Check sheet for the modelled part. Datum: model origin and axes. Units: mm. A direction names the side the tool comes from. Round coordinates to 2 decimals unless told otherwise and drop trailing zeros. Loops run counter-clockwise (first coordinate to the right, second up) from the corner with the lowest first, then second, coordinate; pieces in that order, holes last. Notation, with made-up numbers: M 79,11 L 127,11 A7 ccw 127,23 Z; hole C 81,40.25 d8. An arc over 180 degrees is marked long. Write item = value, one per line. Start each with the question number.
(1) Scan lines: L1, parallel to Y at x = 9, z = 17.5; L2, parallel to Y at x = 6.5, z = 6.5; L3, parallel to Y at x = 0, z = 11. Record each from-to range of solid material in increasing order. Write a range as from..to.
(2) Cross-section at D-D on x = 0. Record the boundary of the cut face in (y, z), plus the area to 3 significant figures.
(3) Cross-section at B-B on y = 15. Record the boundary of the cut face in (x, z), plus the area to 3 significant figures.
(4) Mould release check, pull along X, two halves, no side actions. Record for faces 4 (the face through (26.805, 3.237, 11.586)), 5 (the face through (3.4, 16.4, 11.6)), 6 (the face through (-16.2, 21.6, 11.6)): pulls with the +X half, pulls with the -X half, needs draft (parallel to the pull), parting line crosses it, or undercut.
(5) Set-up check for faces 1 (the face through (-3.399, -16.354, 11.586)), 2 (the face through (12.431, -11.115, 11.586)), 3 (the face through (-16.33, 1.26, 11.59)): record each of +Z, -Z, +X, -X, +Y, -Y from which the full face is reachable in a straight line by a thin tool's end or side.
(6) Go/stop test with flat-tipped pins: P1, Ø2.5, axis at x = 0, y = 0, coming from the +Z side; P2, Ø6, axis at x = -6.5, z = 5, coming from the -Y side; P3, Ø1, axis at x = 16, z = 20, coming from the -Y side; P4, Ø2, axis at x = 12.5, z = 19.5, coming from the +Y side. Record where each tip stops, or that it passes through.
(7) Cross-section at A-A on z = 6.5. Record the boundary of the cut face in (x, y).
(8) Cross-section at C-C on x = 10. Record the boundary of the cut face in (y, z), plus the area to 3 significant figures.
from build123d import *

# Parameters (mm, degrees)
EXTRUDE_1_DEPTH          = 23.5
CUT_EXTRUDE_1_DEPTH      = 45.211198656
CUT_EXTRUDE_1_DEPTH_BACK = 45.211198656
SKETCH_2_R               = 2


with BuildPart() as part:
    # 草图1 → 凸台-拉伸1 (new body)
    with BuildSketch(Plane.XY):
        with BuildLine():
            Line((-18.74404726, 19.433494084), (-5.953134221, 2.483458779))
            Line((-5.953134221, 2.483458779), (-27, 0))
            ThreePointArc((-27, 0), (-26.799738116, -3.282382812), (-26.201923191, -6.516074055))
            Line((-26.201923191, -6.516074055), (-5.228535388, -3.928299208))
            Line((-5.228535388, -3.928299208), (-13.5, -23.382685902))
            ThreePointArc((-13.5, -23.382685902), (-10.557242158, -24.850445429), (-7.457875931, -25.949568139))
            Line((-7.457875931, -25.949568139), (0.77550929, -6.485913341))
            Line((0.77550929, -6.485913341), (13.5, -23.382685902))
            ThreePointArc((13.5, -23.382685902), (16.242495958, -21.568062617), (18.74404726, -19.433494084))
            Line((18.74404726, -19.433494084), (5.938212824, -2.560395934))
            Line((5.938212824, -2.560395934), (27, 0))
            ThreePointArc((27, 0), (26.799738116, 3.282382812), (26.201923191, 6.516074055))
            Line((26.201923191, 6.516074055), (5.200951411, 3.927966656))
            Line((5.200951411, 3.927966656), (13.5, 23.382685902))
            ThreePointArc((13.5, 23.382685902), (10.557242158, 24.850445429), (7.457875931, 25.949568139))
            Line((7.457875931, 25.949568139), (-0.802395418, 6.505702023))
            Line((-0.802395418, 6.505702023), (-13.5, 23.382685902))
            ThreePointArc((-13.5, 23.382685902), (-16.242495958, 21.568062617), (-18.74404726, 19.433494084))
        make_face()
    extrude(amount=EXTRUDE_1_DEPTH)

    # 草图2 → 切除-拉伸1 (cut, two sides: drawn at the far end of the back side and taken through both)
    with BuildSketch(Plane.XY.offset(23.5).offset(-CUT_EXTRUDE_1_DEPTH_BACK)):
        Circle(SKETCH_2_R)
    extrude(amount=CUT_EXTRUDE_1_DEPTH + CUT_EXTRUDE_1_DEPTH_BACK, mode=Mode.SUBTRACT)


solid = part.part
Result:
q1.L1 = -17.41..-6.59, -2.19..4.4, 12.83..25.46
q1.L2 = -14.09..-3.3, -2.49..4.09, 6.97..23.69
q1.L3 = -8.32..-2, 2..8.39
q2.outline = M -8.32,0 L -2,0 L -2,23.5 L -8.32,23.5 Z; M 2,0 L 8.39,0 L 8.39,23.5 L 2,23.5 Z
q2.area = 299 mm^2
q3.outline = M -15.4,0 L -7.19,0 L -7.19,23.5 L -15.4,23.5 Z; M 2.81,0 L 9.92,0 L 9.92,23.5 L 2.81,23.5 Z
q3.area = 360 mm^2
q4.face_4 = pulls with the +X half
q4.face_5 = undercut
q4.face_6 = pulls with the -X half
q5.face_1 = +Z, -Z, -Y
q5.face_2 = +Z, -Z, +X
q5.face_3 = +Z, -Z, -X
q6.P1 = through
q6.P2 = -25.95
q6.P3 = -22.11
q6.P4 = 24.43
q7.outline = M -27,0 A27 ccw -26.2,-6.52 L -5.23,-3.93 L -13.5,-23.38 A27 ccw -7.46,-25.95 L 0.78,-6.49 L 13.5,-23.38 A27 ccw 18.74,-19.43 L 5.94,-2.56 L 27,0 A27 ccw 26.2,6.52 L 5.2,3.93 L 13.5,23.38 A27 ccw 7.46,25.95 L -0.8,6.51 L -13.5,23.38 A27 ccw -18.74,19.43 L -5.95,2.48 Z; hole C 0,0 d4
q8.outline = M -18.74,0 L -7.91,0 L -7.91,23.5 L -18.74,23.5 Z; M -2.07,0 L 4.52,0 L 4.52,23.5 L -2.07,23.5 Z; M 15.18,0 L 25.08,0 L 25.08,23.5 L 15.18,23.5 Z
q8.area = 642 mm^2
